Geometry: final body of the model. Coordinates: model frame, mm. A direction names the side the tool comes from. Give positions to 0.01 mm unless a question says otherwise; leave off trailing zeros. Loops run counter-clockwise (first coordinate to the right, second up) from the corner with the lowest first, then second, coordinate; pieces in that order, holes last. Notation, with made-up numbers: (22.25, 37.5) -> (36.25, 37.5) arc R17 ccw to (36.25, 62.5) -> close; hole circle Ø4 at (66, 32.5). An arc over 180 degrees is marked (long way). One line per question, with ' | ' between items. Start each with the question number.
Item 1: Set-up query: faces 1 (the flat face through (6.5, 7.35, 0.5)), 2 (the flat face through (3, 7.819, -0.5)), 3 (the flat face through (3.94, -1, 1.5)). Return all of +Z, -Z, +X, -X, +Y, -Y with unobstructed straight access to the full face (end or side cutting, diameter ignored); none if empty.
Item 2: Pin query (flat end, axial travel): P1, Ø0.8, axis at x = 6.5, z = 0.5, coming from the +Y side; P2, Ø7, axis at x = -1.5, y = 5.5, coming from the -Z side; P3, Ø0.8, axis at x = -1.5, z = 1.5, coming from the -Y side; P4, Ø2, axis at x = 5, y = 4, coming from the +Z side. Return the tip coordinate at first contact, or that it passes through.
Item 3: Section C-C on z = -0.75. Return loops of the section in (x, y).
Item 4: Mould query, pull axis X, two halves, no side actions, for faces 4 (the flat face through (-6, -0.7, -0.5)), 5 (the flat face through (4.632, -3.2, 1.5)), 6 (the flat face through (3, 8, 2)). Classes: released by +X, released by -X, zero draft, split by the parting line, or undercut.
Item 5: Section D-D on x = 5. Return loops of the section in (y, z).
Item 6: Section A-A on z = 1.6. Return loops of the section in (x, y), then the cut area to 3 significant figures.
Item 7: Material intervals for line 1 along Y through (x, z) = (3.25, 1.5); line 2 along Y through (x, z) = (0.75, 1.5); line 3 along X through (y, z) = (8.25, 1.8), sorted ascending. Write a range as [from, to].
Item 8: Section B-B on y = -6.35. Return loops of the section in (x, z).
from build123d import *

# Parameters (mm, degrees)
SKETCH_1_W          = 14
SKETCH_1_H          = 14.7
EXTRUDE_1_DEPTH     = 1
SKETCH_2_W          = 12
SKETCH_2_H          = 5
EXTRUDE_2_DEPTH     = 1
SKETCH_3_R          = 0.5
CUT_EXTRUDE_1_DEPTH = 2
SKETCH_4_W          = 4.181251824
SKETCH_4_H          = 4.30078239
SKETCH_4_W_2        = 9
SKETCH_4_H_2        = 9
SKETCH_4_W_3        = 1.811721258
SKETCH_4_H_3        = 2.150391195
EXTRUDE_3_DEPTH     = 1
SKETCH_5_W          = 1.98908545
SKETCH_5_H          = 7.5
SKETCH_5_W_2        = 2.470298365
SKETCH_5_H_2        = 2.390611322
EXTRUDE_4_DEPTH     = 1


with BuildPart() as part:
    # 草图1 → 凸台-拉伸1 (new body)
    with BuildSketch(Plane.XY):
        Rectangle(SKETCH_1_W, SKETCH_1_H)
    extrude(amount=EXTRUDE_1_DEPTH)

    # 草图2 → 凸台-拉伸2 (add)
    with BuildSketch(Plane.XY):
        with Locations((0, 9.85)):
            Rectangle(SKETCH_2_W, SKETCH_2_H)
    extrude(amount=EXTRUDE_2_DEPTH)

    # 草图3 → 切除-拉伸1 (cut, through all)
    with BuildSketch(Plane.XY.offset(1)):
        with Locations((-5, 11.35)):
            Circle(SKETCH_3_R)
        with Locations((5, 11.35)):
            Circle(SKETCH_3_R)
        with Locations((-6, -6.35)):
            Circle(SKETCH_3_R)
        with Locations((6, -6.35)):
            Circle(SKETCH_3_R)
    extrude(amount=-CUT_EXTRUDE_1_DEPTH, mode=Mode.SUBTRACT)

    # 草图4 → 凸台-拉伸3 (add)
    with BuildSketch(Plane.XY.offset(1)):
        with Locations((-1.176542894, 8.176542894)):
            Rectangle(SKETCH_4_W, SKETCH_4_H)
        with Locations((-0.560127297, -0.908939121)):
            Rectangle(SKETCH_4_W_2, SKETCH_4_H_2)
        with Locations((3.476926793, 8.336496479)):
            Rectangle(SKETCH_4_W_3, SKETCH_4_H_3)
        with Locations((5.538249561, -3.137858366)):
            Rectangle(SKETCH_4_W_3, SKETCH_4_H_3)
    extrude(amount=EXTRUDE_3_DEPTH)

    # 草图5 → 凸台-拉伸4 (add)
    with BuildSketch(Plane(origin=(0, 0, 0), x_dir=(-1, 0, 0), z_dir=(0, 0, -1))):
        with Locations((5.005457275, -0.6)):
            Rectangle(SKETCH_5_W, SKETCH_5_H)
        with Locations((-2.94842063, 6.623804529)):
            Rectangle(SKETCH_5_W_2, SKETCH_5_H_2)
    extrude(amount=EXTRUDE_4_DEPTH)


solid = part.part
Result sheet:
1) face 1: +Z, -Z, +X, +Y | face 2: -Z, +X, -X, +Y | face 3: +Z, -Y
2) P1: stops at y = 7.35 | P2: stops at z = -1 | P3: stops at y = -5.41 | P4: stops at z = 1
3) outline: (-6, -4.35) -> (-4.01, -4.35) -> (-4.01, 3.15) -> (-6, 3.15) -> close; (1.71, 5.43) -> (4.18, 5.43) -> (4.18, 7.82) -> (1.71, 7.82) -> close
4) face 4: released by -X | face 5: undercut | face 6: zero draft
5) outline: (-7.35, 0) -> (10.85, 0) -> (10.85, 1) -> (-2.06, 1) -> (-2.06, 2) -> (-4.21, 2) -> (-4.21, 1) -> (-7.35, 1) -> close; (11.85, 0) -> (12.35, 0) -> (12.35, 1) -> (11.85, 1) -> close
6) outline: (-5.06, -5.41) -> (3.94, -5.41) -> (3.94, 3.59) -> (-5.06, 3.59) -> close; (-3.27, 6.03) -> (0.91, 6.03) -> (0.91, 10.33) -> (-3.27, 10.33) -> close; (2.57, 7.26) -> (4.38, 7.26) -> (4.38, 9.41) -> (2.57, 9.41) -> close; (4.63, -4.21) -> (6.44, -4.21) -> (6.44, -2.06) -> (4.63, -2.06) -> close | area: 107 mm²
7) line 1: y = [-5.41, 3.59], [7.26, 9.41] | line 2: y = [-5.41, 3.59], [6.03, 10.33] | line 3: x = [-3.27, 0.91], [2.57, 4.38]
8) outline: (-7, 0) -> (-6.5, 0) -> (-6.5, 1) -> (-7, 1) -> close; (-5.5, 0) -> (5.5, 0) -> (5.5, 1) -> (-5.5, 1) -> close; (6.5, 0) -> (7, 0) -> (7, 1) -> (6.5, 1) -> close
